from build123d import *

# Parameters (mm, degrees)
SKETCH2_R           = 14
BOSS_EXTRUDE1_DEPTH = 2
SKETCH3_R           = 2


with BuildPart() as part:
    # Sketch1 → Revolve1 (revolve)
    with BuildSketch(Plane(origin=(0, 0, 0), x_dir=(-1, 0, 0), z_dir=(0, 0, -1)), mode=Mode.PRIVATE) as revolve1_sk:
        with BuildLine():
            Line((-11.972812665, 3.766736765), (-11.972812665, 4.016736765))
            Line((-11.972812665, 4.016736765), (-0.912123334, 4.016736765))
            Line((-0.912123334, 4.016736765), (-0.912123334, 5.466736765))
            Line((-0.912123334, 5.466736765), (-1.912123334, 5.466736765))
            Line((-1.912123334, 5.466736765), (-1.912123334, 5.216736765))
            Line((-1.912123334, 5.216736765), (-12.912123334, 5.216736765))
            ThreePointArc((-12.912123334, 5.216736765), (-13.230357031, 4.328770979), (-12.472812665, 3.766736765))
            Line((-12.472812665, 3.766736765), (-11.972812665, 3.766736765))
        make_face()
    revolve(revolve1_sk.sketch.rotate(Axis((12.175741694, -8.533263235, 0), (-1, 0, 0)), 270), axis=Axis((12.175741694, -8.533263235, 0), (-1, 0, 0)))

    # Sketch2 → Boss-Extrude1 (add)
    with BuildSketch(Plane.ZY.offset(-0.912123334)):
        with Locations((0, -8.533263235)):
            Circle(SKETCH2_R)
    extrude(amount=BOSS_EXTRUDE1_DEPTH)

    # Sweep1: sweep along a path in Sketch4
    with BuildLine(Plane.XY) as sweep1_path:
        Line((-1.087876666, -8.533263235), (-9.087876666, -8.533263235))
        ThreePointArc((-9.087876666, -8.533263235), (-10.502090228, -9.119049673), (-11.087876666, -10.533263235))
        Line((-11.087876666, -10.533263235), (-11.087876666, -17.533263235))
    # Sketch3 → Sweep1 (sweep)
    with BuildSketch(Plane.ZY.offset(1.087876666)):
        with Locations((0, -8.533263235)):
            Circle(SKETCH3_R)
    sweep(path=sweep1_path.line)


solid = part.part
The listing builds one solid part. Answer for the finished solid, in the listing's coordinates (mm). A direction names the side the tool comes from. Coordinates: 2 decimals unless noted, no trailing zeros. Write each loop counter-clockwise with the first axis right and the second up, starting at its lowest first coordinate (ties: lowest second). Pieces come first, ordered by that corner, then holes. Notation, with made-up numbers: M -27,67 L 14,67 A16 ccw 14,89 Z; hole C 32.25,68.25 d2. An arc over 180 degrees is marked long. Put each result on its own line as item: value. Start each with the question number.
1. Consider line 1 (Y direction, x = 12.2, z = 0); line 2 (X direction, y = -10.5, z = 8); line 3 (Z direction, x = 8.75, y = -7.25). Determine where each line is inside the solid, lowest interval first. Write a range as from..to.
2. Which of the six approach directions +Z, -Z, +X, -X, +Y, -Y give full straight-line access (tool end or side, diameter ignored) to faces 1 (the cylindrical face through (0.43, -22.2, -3.03)), 2 (the cylindrical face through (-5.144, -10.486, -0.434)), 3 (the cylindrical face through (7.5, 5.1, -1.8))?
3. Flat-ended cylindrical pins translate along their axes: P1, Ø7.5, axis at y = -11.5, z = 1, coming from the -X side; P2, Ø8, axis at x = 9, y = 0, coming from the -Z side; P3, Ø10, axis at x = 7.5, y = -1.5, coming from the +Z side; P4, Ø7.5, axis at y = -14.5, z = -5, coming from the +X side. Find the tip coordinate at first contact, or state that the pin passes through.
4. For a pull along Y with two mould halves and no side action, classify faces 4 (the flat face through (-11, -17.533, 0)), 5 (the cylindrical face through (6.37, -4.76, 11.97)), 6 (the cylindrical face through (12.219, -19.445, 5.676)), 7 (the cylindrical face through (-13.07, -14.08, -0.26)) as pulls with the +Y half, pulls with the -Y half, needs draft (parallel to the pull), parting line crosses it, or undercut.
5. A cutting plane is placed at A-A on x = 4.75. Write down the section's boundary in (y, z), then the cut area to 3 significant figures.
Resolved:
1. line 1: y = -22.28..-20.83, 3.77..5.22
1. line 2: x = -1.09..0.91
1. line 3: z = -13.69..-12.48, 12.48..13.69
2. face 1: +X, -X
2. face 2: none
2. face 3: +X
3. P1: stops at x = -13.09
3. P2: stops at z = -12.98
3. P3: stops at z = 13.6
3. P4: stops at x = 0.91
4. face 4: pulls with the -Y half
4. face 5: undercut
4. face 6: undercut
4. face 7: needs draft
5. outline: C -8.53,0 d27.5; hole C -8.53,0 d25.1
5. area: 99.1 mm2
